```python
from build123d import *

# Parameters (mm, degrees)
SKETCH1_W      = 35.56
SKETCH1_H      = 17.78
BOARD_DEPTH    = 1.57
SKETCH2_W      = 5
SKETCH2_H      = 8.06
MICROUSB_DEPTH = 2.5
SKETCH3_W      = 2.2
SKETCH3_H      = 3.1
BUTTON_DEPTH   = 2.5


with BuildPart() as part:
    # Sketch1 → Board (new body)
    with BuildSketch(Plane(origin=(0, 0, 0), x_dir=(1, 0, 0), z_dir=(0, 1, 0))):
        Rectangle(SKETCH1_W, SKETCH1_H)
    extrude(amount=BOARD_DEPTH)

    # Sketch2 → MicroUSB (add)
    with BuildSketch(Plane(origin=(0, 1.57, 0), x_dir=(1, 0, 0), z_dir=(0, 1, 0))):
        with Locations((-15.28, 0)):
            Rectangle(SKETCH2_W, SKETCH2_H)
    extrude(amount=MICROUSB_DEPTH)

    # Sketch3 → Button (add)
    with BuildSketch(Plane(origin=(0, 1.57, 0), x_dir=(1, 0, 0), z_dir=(0, 1, 0))):
        with Locations((12.19, 0)):
            Rectangle(SKETCH3_W, SKETCH3_H)
    extrude(amount=BUTTON_DEPTH)


solid = part.part
```
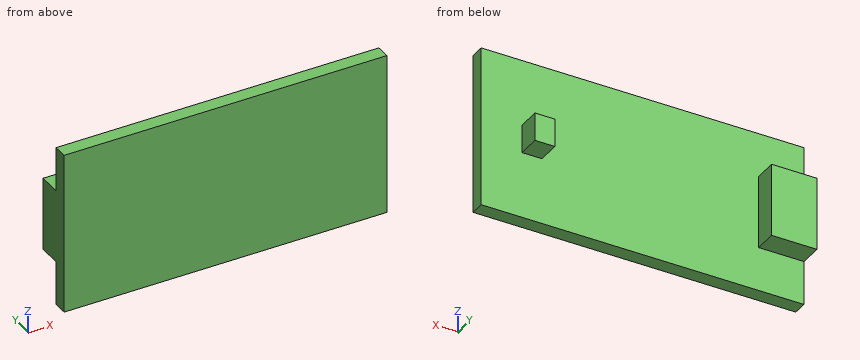
Read the model definition and answer for the solid it produces. Units are mm, in the model's axes. Give positions to 0.01 mm unless a question says otherwise; leave off trailing zeros. Loops run counter-clockwise (first coordinate to the right, second up) from the corner with the lowest first, then second, coordinate; pieces in that order, holes last.
Item 1: The part is cut by section B-B (x = 3). Write down the section's boundary in (y, z).
Item 2: Find the intervals of material crossed by line 1 along X through (y, z) = (3.05, -1.5); line 2 along Y through (x, z) = (-3, -0.5); line 3 along X through (y, z) = (2.7, -3.5), in increasing order.
Item 3: The part is cut by section C-C (z = 7.75). Write down the section's boundary in (x, y).
Item 4: The part is cut by section A-A (z = -1). Write down the section's boundary in (x, y), and give its area (3 significant figures).
Item 5: Each of these flat-tipped pins is pushed along its axis until it touches: pin 1 Ø1.2 at (x, y) = (-16.5, 3) entering from +Z; pin 2 Ø2 at (x, y) = (-16, 3) entering from -Z; pin 3 Ø5 at (x, z) = (1.5, 3) entering from +Y. Where does it stop, or does it pass through?
Taken from the geometry:
1. outline: (0, -8.89) - (1.57, -8.89) - (1.57, 8.89) - (0, 8.89) - close
2. line 1: x = -17.78 to -12.78, 11.09 to 13.29
2. line 2: y = 0 to 1.57
2. line 3: x = -17.78 to -12.78
3. outline: (-17.78, 0) - (17.78, 0) - (17.78, 1.57) - (-17.78, 1.57) - close
4. outline: (-17.78, 0) - (17.78, 0) - (17.78, 1.57) - (13.29, 1.57) - (13.29, 4.07) - (11.09, 4.07) - (11.09, 1.57) - (-12.78, 1.57) - (-12.78, 4.07) - (-17.78, 4.07) - close
4. area: 73.8 mm2
5. pin 1: stops at z = 4.03
5. pin 2: stops at z = -4.03
5. pin 3: stops at y = 1.57
